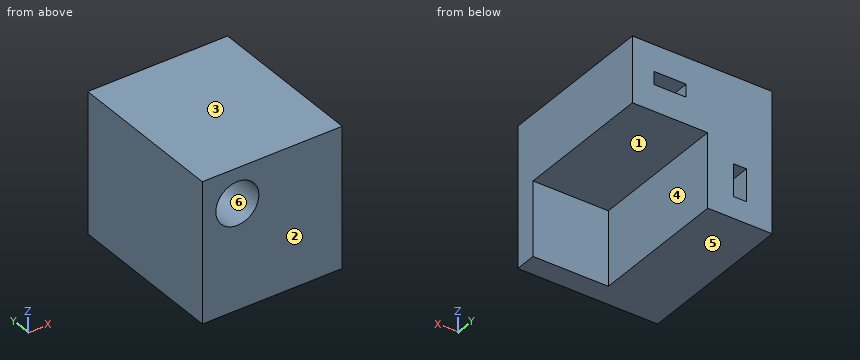
```python
from build123d import *

# Parameters (mm, degrees)
SKETCH3_W           = 16.51
SKETCH3_H           = 16.51
BOSS_EXTRUDE2_DEPTH = 19.05
SKETCH5_R           = 2.54
CUT_EXTRUDE2_DEPTH  = 5.715
SKETCH6_W           = 8.89
SKETCH6_H           = 8.765916865
CUT_EXTRUDE3_DEPTH  = 16.51
SKETCH7_W           = 1.524
SKETCH7_H           = 3.81
SKETCH7_W_2         = 3.81
SKETCH7_H_2         = 1.524
CUT_EXTRUDE4_DEPTH  = 2.54


with BuildPart() as part:
    # Sketch3 → Boss-Extrude2 (new body)
    with BuildSketch(Plane(origin=(0, 0, 0), x_dir=(1, 0, 0), z_dir=(0, 1, 0))):
        Rectangle(SKETCH3_W, SKETCH3_H)
    extrude(amount=BOSS_EXTRUDE2_DEPTH)

    # Sketch5 → Cut-Extrude2 (cut)
    with BuildSketch(Plane.XZ):
        with Locations(Location((-4.1275, 4.1275, 0), (0, 0, 270))):
            Circle(SKETCH5_R)
    extrude(amount=-CUT_EXTRUDE2_DEPTH, mode=Mode.SUBTRACT)

    # Sketch6 → Cut-Extrude3 (cut)
    with BuildSketch(Plane(origin=(0, 19.05, 0), x_dir=(1, 0, 0), z_dir=(0, 1, 0))):
        with Locations((3.81, 3.872041568)):
            Rectangle(SKETCH6_W, SKETCH6_H)
    extrude(amount=-CUT_EXTRUDE3_DEPTH, mode=Mode.SUBTRACT)

    # Sketch7 → Cut-Extrude4 (cut)
    with BuildSketch(Plane(origin=(0, 19.05, 0), x_dir=(1, 0, 0), z_dir=(0, 1, 0))):
        with Locations((-4.445, 3.81)):
            Rectangle(SKETCH7_W, SKETCH7_H)
        with Locations((3.81, -4.382958433)):
            Rectangle(SKETCH7_W_2, SKETCH7_H_2)
    extrude(amount=-CUT_EXTRUDE4_DEPTH, mode=Mode.SUBTRACT)


solid = part.part
```
Input: part model. Units: mm. Frame: model coordinates. Face numbers are marked on the shaded views. A direction names the side the tool comes from. Give positions to 0.01 mm unless a question says otherwise; leave off trailing zeros. Order: outer loops, then holes, each group sorted by start corner. A loop starts at its lowest first (then second) coordinate and runs counter-clockwise, first axis right, second up. Notation, with made-up numbers: M 85,6 L 104,6 A5 cw 104,12 Z; hole C 86.5,44.25 d9. An arc over 180 degrees is marked long. One line per question, with ' | ' between items.
1) Section C-C on x = 3. Output: boundary loops of the cut face in (y, z) (3 decimals), and give its area (3 significant figures).
Filled in:
outline: M 0,-8.255 L 2.54,-8.255 L 2.54,0.511 L 19.05,0.511 L 19.05,3.621 L 16.51,3.621 L 16.51,5.145 L 19.05,5.145 L 19.05,8.255 L 0,8.255 Z | area: 166 mm2
2) Access query for the marked faces 1 and 2. Directions: +Z, -Z, +X, -X, +Y, -Y. A direction counts if a zero-diameter tool reaches every point of the face in a straight line with its end or side. Return the directions, or none.
Filled in:
face 1: -Z, +X, +Y | face 2: +Z, -Z, +X, -X, -Y
3) Section D-D on y = 15.5. Output: boundary loops of the cut face in (x, z) (3 decimals), and give its area (3 significant figures).
Filled in:
outline: M -8.255,-8.255 L -0.635,-8.255 L -0.635,0.511 L 8.255,0.511 L 8.255,8.255 L -8.255,8.255 Z | area: 195 mm2
4) Ray query, L1, parallel to Z at x = 1, y = 8 (3 decimals); L2, parallel to X at y = 11.75, z = -3 (3 decimals); L3, parallel to Y at x = 6.5, z = -6.25. Return the intervals inside material, ascending.
Filled in:
L1: z = 0.511 to 8.255 | L2: x = -8.255 to -0.635 | L3: y = 0 to 2.54
5) Contact query for flat-ended pins moving along their axis: P1, Ø0.8, axis at x = 3, z = 4.5, coming from the +Y side; P2, Ø9.5, axis at y = 14, z = -5.5, coming from the +X side (3 decimals); P3, Ø2, axis at x = 3.5, y = 17.5, coming from the -Z side. Output: stop coordinate, or through.
Filled in:
P1: stops at y = 16.51 | P2: stops at x = -0.635 | P3: stops at z = 0.51
6) Section A-A on y = 17.75. Output: boundary loops of the cut face in (x, z) (3 decimals), and give its area (3 significant figures).
Filled in:
outline: M -8.255,-8.255 L -0.635,-8.255 L -0.635,0.511 L 8.255,0.511 L 8.255,8.255 L -8.255,8.255 Z; hole M -5.207,-5.715 L -3.683,-5.715 L -3.683,-1.905 L -5.207,-1.905 Z; hole M 1.905,3.621 L 5.715,3.621 L 5.715,5.145 L 1.905,5.145 Z | area: 183 mm2
7) Draft query along Z for the marked faces 3, 4, 5 and 6. Return one class per face: pulls with the +Z half, pulls with the -Z half, needs draft (parallel to the pull), parting line crosses it, or undercut.
Filled in:
face 3: pulls with the +Z half | face 4: needs draft | face 5: pulls with the -Z half | face 6: undercut
8) Section B-B on z = -0.25. Output: boundary loops of the cut face in (x, y) (3 decimals).
Filled in:
outline: M -8.255,0 L 8.255,0 L 8.255,2.54 L -0.635,2.54 L -0.635,19.05 L -8.255,19.05 Z
